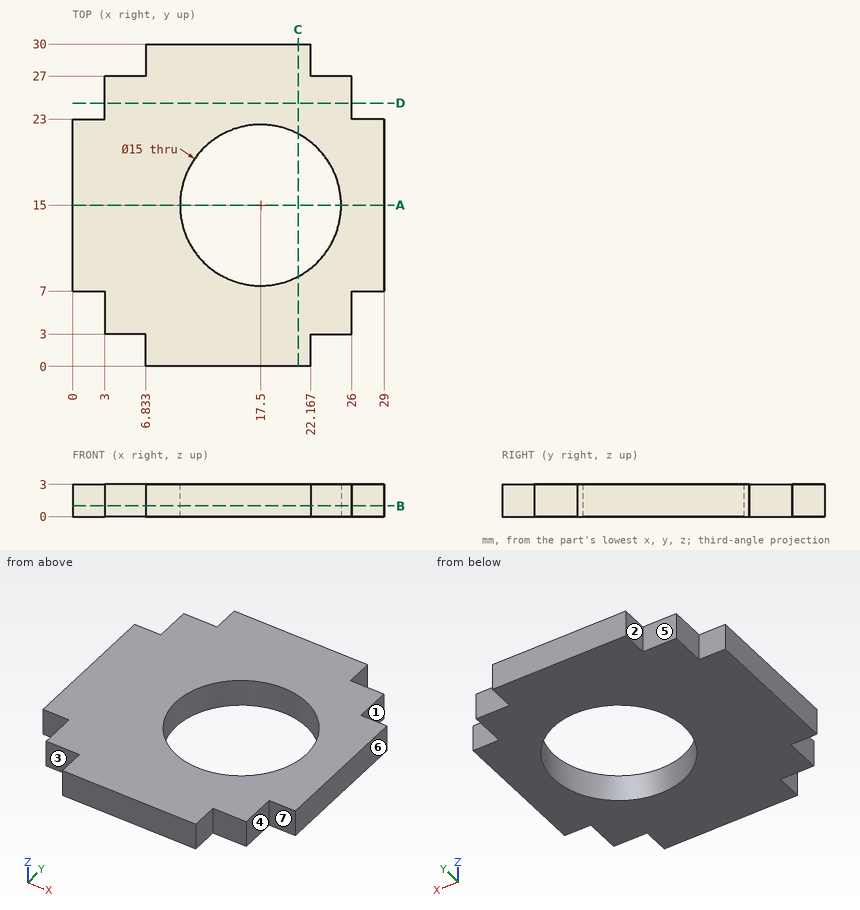
The figure shows three views and two pictorial views of one solid part (mm, origin at its lowest corner). Answer the questions. A direction names the side the tool comes from. Give positions to 0.01 mm unless a question says otherwise; leave off trailing zeros. Order: outer loops, then holes, each group sorted by start corner. A loop starts at its lowest first (then second) coordinate and runs counter-clockwise, first axis right, second up. Notation, with made-up numbers: (18, 36) -> (53, 36) arc R17 cw to (53, 53) -> close; hole circle Ø8 at (43.25, 42.5). An arc over 180 degrees is marked (long way). One line per item, written item: value.
1) Find section A-A, the plane y = 15. Determine the outline of the cut face in (x, z), plus the area to 3 significant figures.
Reported:
outline: (0, 0) -> (10, 0) -> (10, 3) -> (0, 3) -> close; (25, 0) -> (29, 0) -> (29, 3) -> (25, 3) -> close
area: 42.0 mm^2
2) Flat-ended cylindrical pins translate along their axes: P1, Ø1.5, axis at y = 26, z = 2, coming from the -X side; P2, Ø1.5, axis at y = 25, z = 1.5, coming from the +X side; P3, Ø0.9, axis at y = 28.5, z = 1.5, coming from the +X side. Find the tip coordinate at first contact, or state that the pin passes through.
Reported:
P1: stops at x = 3
P2: stops at x = 26
P3: stops at x = 22.17
3) Find section B-B, the plane z = 1. Determine the outline of the cut face in (x, y), plus the area to 3 significant figures.
Reported:
outline: (0, 7) -> (3, 7) -> (3, 3) -> (6.83, 3) -> (6.83, 0) -> (22.17, 0) -> (22.17, 3) -> (26, 3) -> (26, 7) -> (29, 7) -> (29, 23) -> (26, 23) -> (26, 27) -> (22.17, 27) -> (22.17, 30) -> (6.83, 30) -> (6.83, 27) -> (3, 27) -> (3, 23) -> (0, 23) -> close; hole circle Ø15 at (17.5, 15)
area: 563 mm^2
4) Find the intervals of material crossed by line 1 (Y direction, x = 3.75, z = 2.3); line 2 (X direction, y = 21.5, z = 2.3) (1 decimal); line 3 (Y direction, x = 12, z = 1), in increasing order.
Reported:
line 1: y = 3 to 27
line 2: x = 0 to 13.8, 21.2 to 29
line 3: y = 0 to 9.9, 20.1 to 30
5) Find section D-D, the plane y = 24.5. Determine the outline of the cut face in (x, z), plus the area to 3 significant figures.
Reported:
outline: (3, 0) -> (26, 0) -> (26, 3) -> (3, 3) -> close
area: 69.0 mm^2
6) Find section C-C, the plane x = 21. Determine the outline of the cut face in (y, z), plus the area to 3 significant figures.
Reported:
outline: (0, 0) -> (8.37, 0) -> (8.37, 3) -> (0, 3) -> close; (21.63, 0) -> (30, 0) -> (30, 3) -> (21.63, 3) -> close
area: 50.2 mm^2
7) A tool of negligible diameter and unlimited length cuts with its end or side. For the marked faces 1, 2, 3 and 4, from which of +Z, -Z, +X, -X, +Y, -Y can it reach the whole face along a straight path? Write none if from no direction.
Reported:
face 1: +Z, -Z, +X, +Y
face 2: +Z, -Z, -X, +Y
face 3: +Z, -Z, -X, -Y
face 4: +Z, -Z, +X, -Y
8) Determine the mould class of the marked faces 5, 6 and 7 for opening direction Y: pulls with the +Y half, pulls with the -Y half, needs draft (parallel to the pull), parting line crosses it, or undercut.
Reported:
face 5: pulls with the +Y half
face 6: needs draft
face 7: pulls with the -Y half
